Build history of the part. All positions in model axes, mm. Face numbers are marked on the shaded views. Give positions to 0.01 mm unless a question says otherwise; leave off trailing zeros. Write each loop counter-clockwise with the first axis right and the second up, starting at its lowest first coordinate (ties: lowest second). Pieces come first, ordered by that corner, then holes. Notation, with made-up numbers: M 35.25,68.5 L 70.25,68.5 A21 cw 70.25,75.5 Z; hole C -20,-5.5 d8. An arc over 180 degrees is marked long. Return JSON: item names as keys, results as strings. Group by question number.
Q1. Wall check: probe 1 along Y at (x, z) = (-25, 4). Give the ranges that are in metal, low to high.
Q2. Band-saw the part on A-A, the plane y = -25. Give the cut face in (x, z).
Q3. Pull direction Z, two halves, no side cores. Call the marked faces 1 and 2: +Z half, -Z half, draft (parallel to the pull), parting line (faces both ways), or undercut.
Q4. Band-saw the part on C-C, the plane z = 2.5. Give the cut face in (x, y).
from build123d import *

# Parameters (mm, degrees)
SKETCH1_W                = 75
SKETCH1_H                = 75
BOSS_EXTRUDE1_DEPTH      = 5
F_7_0_7_DIAMETER_HOLE1_D = 7
FILLET1_R                = 10


with BuildPart() as part:
    # Sketch1 → Boss-Extrude1 (new body)
    with BuildSketch(Plane.XY):
        Rectangle(SKETCH1_W, SKETCH1_H)
    extrude(amount=BOSS_EXTRUDE1_DEPTH)

    # Ø7.0 (7) Diameter Hole1 (through all)
    with Locations(Plane.XY.offset(5)):
        with Locations((-25, 25), (-25, -25), (25, -25), (25, 25)):
            Hole(F_7_0_7_DIAMETER_HOLE1_D / 2)

    # Fillet1
    fillet1_edges = [part.edges().sort_by_distance(p)[0] for p in [
        (-37.5, 37.5, 2.5),
        (37.5, 37.5, 2.5),
        (37.5, -37.5, 2.5),
        (-37.5, -37.5, 2.5),
    ]]
    fillet(fillet1_edges, radius=FILLET1_R)


solid = part.part
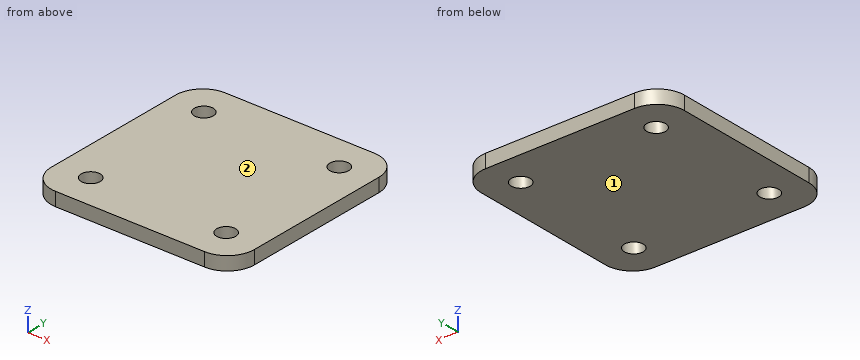
From the geometry:
{
 "1": {"probe 1": "y = -37.5 to -28.5, -21.5 to 21.5, 28.5 to 37.5"},
 "2": {"outline": "M -37.5,0 L -28.5,0 L -28.5,5 L -37.5,5 Z; M -21.5,0 L 21.5,0 L 21.5,5 L -21.5,5 Z; M 28.5,0 L 37.5,0 L 37.5,5 L 28.5,5 Z"},
 "3": {"face 1": "-Z half", "face 2": "+Z half"},
 "4": {"outline": "M -37.5,-27.5 A10 ccw -27.5,-37.5 L 27.5,-37.5 A10 ccw 37.5,-27.5 L 37.5,27.5 A10 ccw 27.5,37.5 L -27.5,37.5 A10 ccw -37.5,27.5 Z; hole C -25,-25 d7; hole C -25,25 d7; hole C 25,-25 d7; hole C 25,25 d7"}
}
